Input: dimensioned drawing with shaded views. Units: mm. Origin: part minimum x, y, z. Coordinates: 2 decimals unless noted, no trailing zeros. Loops run counter-clockwise (first coordinate to the right, second up) from the corner with the lowest first, then second, coordinate; pieces in that order, holes last.
Item 1: Section B-B on y = 1. Return loops of the section in (x, z).
Item 2: Section A-A on z = 4.25. Return loops of the section in (x, y), and give its area (3 significant figures).
Item 3: Section D-D on z = 6.5. Return loops of the section in (x, y).
Item 4: Contact query for a flat-ended pin moving along its axis: P1, Ø1, axis at x = 1.5, z = 4, coming from the -Y side (1 decimal). Output: stop coordinate, or through.
Item 5: Ray query, line 1 along Y through (x, z) = (0.65, 1); line 2 along Z through (x, y) = (1.6, 1.5); line 3 along Y through (x, z) = (2.3, 3.5) (1 decimal). Return the intervals inside material, ascending.
Item 6: Section C-C on x = 2.15. Return loops of the section in (y, z).
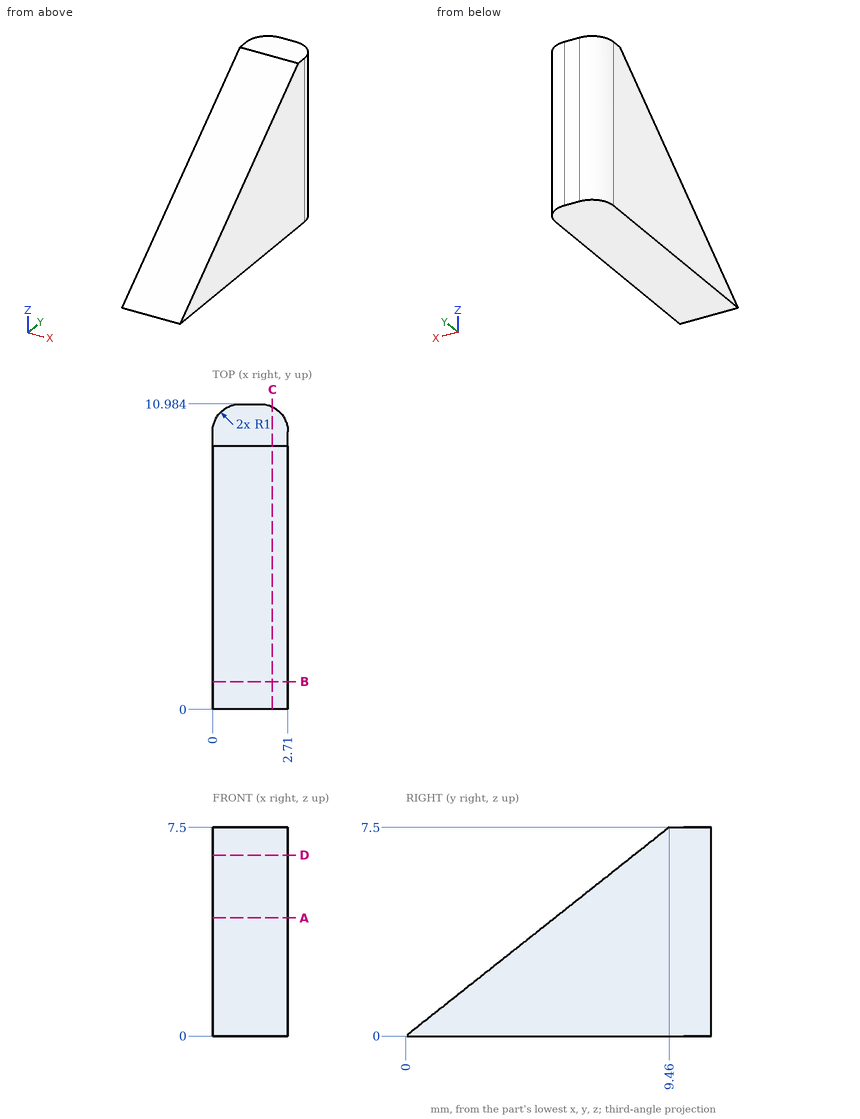
Results found:
1. outline: (0, 0) - (2.71, 0) - (2.71, 0.79) - (0, 0.79) - close
2. outline: (0, 5.36) - (2.71, 5.36) - (2.71, 9.98) arc R1 ccw to (1.71, 10.98) - (1, 10.98) arc R1 ccw to (0, 9.98) - close
2. area: 14.8 mm2
3. outline: (0, 8.2) - (2.71, 8.2) - (2.71, 9.98) arc R1 ccw to (1.71, 10.98) - (1, 10.98) arc R1 ccw to (0, 9.98) - close
4. P1: stops at y = 4.4
5. line 1: y = 1.26 to 10.92
5. line 2: z = 0 to 1.19
5. line 3: y = 4.4 to 10.8
6. outline: (0, 0) - (10.88, 0) - (10.88, 7.5) - (9.46, 7.5) - close
